```python
from build123d import *

# Parameters (mm, degrees)
SKETCH1_W           = 120
SKETCH1_H           = 120
BOSS_EXTRUDE2_DEPTH = 130
SKETCH20_W          = 12
SKETCH20_H          = 21.5
CUT_EXTRUDE3_DEPTH  = 33
SKETCH10_W          = 12
SKETCH10_H          = 8
CUT_EXTRUDE4_DEPTH  = 91
SKETCH2_R           = 18.5
CUT_EXTRUDE5_DEPTH  = 32.5
SKETCH24_W          = 15
SKETCH24_H          = 15
BOSS_EXTRUDE4_DEPTH = 20
SKETCH16_W          = 20
SKETCH16_H          = 20
BOSS_EXTRUDE5_DEPTH = 20
SKETCH27_W          = 15
SKETCH27_H          = 15
BOSS_EXTRUDE6_DEPTH = 20
SKETCH28_W          = 15
SKETCH28_H          = 15
BOSS_EXTRUDE7_DEPTH = 20
SKETCH29_W          = 15
SKETCH29_H          = 15
BOSS_EXTRUDE8_DEPTH = 20
CHAMFER3_SIZE       = 5
SKETCH38_W          = 13
SKETCH38_H          = 32.5
CUT_EXTRUDE7_DEPTH  = 30
CHAMFER4_SIZE       = 5


with BuildPart() as part:
    # Sketch1 → Boss-Extrude2 (new body)
    with BuildSketch(Plane.XY):
        with Locations((60, 60)):
            Rectangle(SKETCH1_W, SKETCH1_H)
    extrude(amount=-BOSS_EXTRUDE2_DEPTH)

    # Sketch20 → Cut-Extrude3 (cut)
    with BuildSketch(Plane(origin=(0, 0, -130), x_dir=(-1, 0, 0), z_dir=(0, 0, -1))):
        with Locations((-60, 28.25)):
            Rectangle(SKETCH20_W, SKETCH20_H)
    extrude(amount=-CUT_EXTRUDE3_DEPTH, mode=Mode.SUBTRACT)

    # Sketch10 → Cut-Extrude4 (cut)
    with BuildSketch(Plane(origin=(0, 120, 0), x_dir=(1, 0, 0), z_dir=(0, 1, 0))):
        with Locations((60, 101)):
            Rectangle(SKETCH10_W, SKETCH10_H)
    extrude(amount=-CUT_EXTRUDE4_DEPTH, mode=Mode.SUBTRACT)

    # Sketch2 → Cut-Extrude5 (cut)
    with BuildSketch(Plane.XY):
        with Locations((60, 91.5)):
            Circle(SKETCH2_R)
    extrude(amount=-CUT_EXTRUDE5_DEPTH, mode=Mode.SUBTRACT)

    # Sketch24 → Boss-Extrude4 (add)
    with BuildSketch(Plane(origin=(0, 120, 0), x_dir=(1, 0, 0), z_dir=(0, 1, 0))):
        with Locations((7.5, 122.5)):
            Rectangle(SKETCH24_W, SKETCH24_H)
    extrude(amount=BOSS_EXTRUDE4_DEPTH)

    # Sketch16 → Boss-Extrude5 (add)
    with BuildSketch(Plane(origin=(0, 120, 0), x_dir=(1, 0, 0), z_dir=(0, 1, 0))):
        with Locations((60, 65)):
            Rectangle(SKETCH16_W, SKETCH16_H)
    extrude(amount=BOSS_EXTRUDE5_DEPTH)

    # Sketch27 → Boss-Extrude6 (add)
    with BuildSketch(Plane(origin=(0, 120, 0), x_dir=(1, 0, 0), z_dir=(0, 1, 0))):
        with Locations((7.5, 7.5)):
            Rectangle(SKETCH27_W, SKETCH27_H)
    extrude(amount=BOSS_EXTRUDE6_DEPTH)

    # Sketch28 → Boss-Extrude7 (add)
    with BuildSketch(Plane(origin=(0, 120, 0), x_dir=(1, 0, 0), z_dir=(0, 1, 0))):
        with Locations((112.5, 122.5)):
            Rectangle(SKETCH28_W, SKETCH28_H)
    extrude(amount=BOSS_EXTRUDE7_DEPTH)

    # Sketch29 → Boss-Extrude8 (add)
    with BuildSketch(Plane(origin=(0, 120, 0), x_dir=(1, 0, 0), z_dir=(0, 1, 0))):
        with Locations((112.5, 7.5)):
            Rectangle(SKETCH29_W, SKETCH29_H)
    extrude(amount=BOSS_EXTRUDE8_DEPTH)

    # Chamfer3
    chamfer3_edges = [part.edges().sort_by_distance(p)[0] for p in [
        (60, 120, -105),
        (66, 120, -101),
        (54, 120, -101),
        (60, 120, -97),
    ]]
    chamfer(chamfer3_edges, length=CHAMFER3_SIZE)

    # Sketch38 → Cut-Extrude7 (cut)
    with BuildSketch(Plane(origin=(0, 120, 0), x_dir=(1, 0, 0), z_dir=(0, 1, 0))):
        with Locations((60, 16.25)):
            Rectangle(SKETCH38_W, SKETCH38_H)
    extrude(amount=-CUT_EXTRUDE7_DEPTH, mode=Mode.SUBTRACT)

    # Chamfer4
    chamfer4_edges = [part.edges().sort_by_distance(p)[0] for p in [
        (120, 120, -65),
        (85.75, 120, 0),
        (60, 120, -130),
        (0, 120, -65),
        (34.25, 120, 0),
    ]]
    chamfer(chamfer4_edges, length=CHAMFER4_SIZE)


solid = part.part
```
Work out the finished part from the listing and answer in its coordinate system (mm). A direction names the side the tool comes from. Round coordinates to 2 decimals unless told otherwise and drop trailing zeros. Write each loop counter-clockwise with the first axis right and the second up, starting at its lowest first coordinate (ties: lowest second). Pieces come first, ordered by that corner, then holes. Notation, with made-up numbers: (51.5, 75) -> (64.5, 75) arc R23 ccw to (64.5, 85) -> close; hole circle Ø2 at (41.25, -31). An arc over 180 degrees is marked (long way). Write each question's results on one line, items separated by ' | '.
1) The part is cut by section A-A (x = 60). Write down the section's boundary in (y, z), and give its area (3 significant figures).
Findings:
outline: (0, -130) -> (17.5, -130) -> (17.5, -97) -> (115, -97) -> (120, -92) -> (120, -75) -> (140, -75) -> (140, -55) -> (120, -55) -> (120, -32.5) -> (73, -32.5) -> (73, 0) -> (0, 0) -> close; (39, -130) -> (115, -130) -> (120, -125) -> (120, -110) -> (115, -105) -> (39, -105) -> close | area: 13,100 mm²
2) For a pull along Z with two mould halves and no side action, classify faces 5 (the flat face through (2, 117, -64)), 6 (the flat face through (60, 130, -55)), 7 (the flat face through (112, 140, -123)), 8 (the flat face through (60, 67, -97)) as +Z half, -Z half, draft (parallel to the pull), parting line (faces both ways), or undercut.
Findings:
face 5: undercut | face 6: +Z half | face 7: draft | face 8: undercut
3) The part is cut by section B-B (y = 91.5). Write down the section's boundary in (x, z).
Findings:
outline: (0, -130) -> (120, -130) -> (120, 0) -> (78.5, 0) -> (78.5, -32.5) -> (41.5, -32.5) -> (41.5, 0) -> (0, 0) -> close; hole (54, -105) -> (66, -105) -> (66, -97) -> (54, -97) -> close
4) The part is cut by section C-C (y = 37). Write down the section's boundary in (x, z).
Findings:
outline: (0, -130) -> (54, -130) -> (54, -97) -> (66, -97) -> (66, -130) -> (120, -130) -> (120, 0) -> (0, 0) -> close
5) The part is cut by section D-D (z = -63). Write down the section's boundary in (x, y), and give its area (3 significant figures).
Findings:
outline: (0, 0) -> (120, 0) -> (120, 115) -> (115, 120) -> (70, 120) -> (70, 140) -> (50, 140) -> (50, 120) -> (5, 120) -> (0, 115) -> close | area: 14,800 mm²
6) Which of the six approach directions +Z, -Z, +X, -X, +Y, -Y give full straight-line access (tool end or side, diameter ignored) to faces 1 (the flat face through (54, 45, -102)), 2 (the flat face through (85, 117, -2)), 3 (the flat face through (59, 118, -127)), 4 (the cylindrical face through (59.279, 73.014, -16.022))?
Findings:
face 1: none | face 2: +Z, +Y | face 3: -Z, +Y | face 4: +Z
7) Flat-ended cylindrical pins translate along their axes: pin 1 (12 mm diameter, centred on y = 127, z = -5, fed in from -X); pin 2 (10 mm diameter, centred on y = 125.5, z = -60.5, fed in from -X); pin 3 (22 mm diameter, centred on x = 60.5, y = 131.5, fed in from -Z); pin 4 (6 mm diameter, centred on x = 62.5, z = -118, fed in from +Y). Find the tip coordinate at first contact, or state that the pin passes through.
Findings:
pin 1: stops at x = 0 | pin 2: stops at x = 50 | pin 3: stops at z = -75 | pin 4: stops at y = 120
8) Consider line 1 along X through (y, z) = (91.5, -6.5); line 2 along X through (y, z) = (123, -11.5); line 3 along Z through (x, y) = (64.5, 61). Determine where each line is inside the solid, lowest interval first. Write a range as [from, to].
Findings:
line 1: x = [0, 41.5], [78.5, 120] | line 2: x = [0, 15], [105, 120] | line 3: z = [-130, -105], [-97, 0]
